Geometry check sheet. Reference: the model listing, model coordinates, mm. A direction names the side the tool comes from. Round coordinates to 2 decimals unless told otherwise and drop trailing zeros. Write each loop counter-clockwise with the first axis right and the second up, starting at its lowest first coordinate (ties: lowest second). Pieces come first, ordered by that corner, then holes. Notation, with made-up numbers: M 1,-13.5 L 39,-13.5 A25 ccw 39,19.5 Z; hole C 73,63 d2. An arc over 180 degrees is marked long. Use a Markdown table: item, result.
```python
from build123d import *
from build123d.topology import SkipClean

# Parameters (mm, degrees)
SKETCH_1_W            = 9.1
SKETCH_1_H            = 5.6
EXTRUDE_1_DEPTH       = 1.78
SKETCH_2_W            = 6.1
SKETCH_2_H            = 5.6
EXTRUDE_2_DEPTH       = 1.4
SWEEP_START           = -2.28
SWEEP_2_DEPTH         = 0.76
MIRROR_START          = -2.28
MIRROR_2_COPY_1_DEPTH = 0.76


# Read off the part's stored shape, not the designer's step: 스윕2
with BuildPart() as part:
    # 스케치1 → 보스-돌출1 (new body)
    with BuildSketch(Plane.XY):
        Rectangle(SKETCH_1_W, SKETCH_1_H)
    extrude(amount=EXTRUDE_1_DEPTH)

    # 스케치2 → 보스-돌출2 (add)
    with BuildSketch(Plane.XY.offset(1.78)):
        Rectangle(SKETCH_2_W, SKETCH_2_H)
    extrude(amount=EXTRUDE_2_DEPTH)

    # 스케치3 → 회전1 (revolve)
    with SkipClean():  # the faces are left unmerged after this step: merging them gives an invalid solid
        with BuildSketch(Plane(origin=(0, 0, 0), x_dir=(1, 0, 0), z_dir=(0, 1, 0))):
            with BuildLine():
                Line((-0.579062876, -3.18), (0.579062876, -3.18))
                ThreePointArc((0.579062876, -3.18), (0, -3.759062876), (-0.579062876, -3.18))
            make_face()
        revolve(axis=Axis((-0.579062876, 0, 3.18), (1, 0, 0)))

    # 스윕2 outline → 스윕2 (add)
    with SkipClean():  # the faces are left unmerged after this step: merging them gives an invalid solid
        with BuildSketch(Plane(origin=(0, 0, 0), x_dir=(1, 0, 0), z_dir=(0, 1, 0)).offset(SWEEP_START)):
            with BuildLine():
                Line((6.848797328, -0.399996384), (6.851202672, -3.616e-06))
                Line((6.851202672, -3.616e-06), (6.043424326, 0.004853607))
                ThreePointArc((6.043424326, 0.004853607), (5.654230205, -0.155982007), (5.492969053, -0.545))
                ThreePointArc((5.492969053, -0.545), (5.450499536, -0.647530483), (5.347969053, -0.69))
                Line((5.347969053, -0.69), (4.55, -0.69))
                Line((4.55, -0.69), (4.55, -1.09))
                Line((4.55, -1.09), (5.347969053, -1.09))
                ThreePointArc((5.347969053, -1.09), (5.733342249, -0.930373196), (5.892969053, -0.545))
                ThreePointArc((5.892969053, -0.545), (5.936647868, -0.439250079), (6.042221667, -0.395147271))
                Line((6.042221667, -0.395147271), (6.848797328, -0.399996384))
            make_face()
        sweep_2 = extrude(amount=SWEEP_2_DEPTH)

    # 대칭 복사1: 스윕2 across plane
    with SkipClean():  # the faces are left unmerged after this step: merging them gives an invalid solid
        add(sweep_2.mirror(Plane.ZX))

    # 대칭 복사2: 스윕2 across plane
    with SkipClean():  # the faces are left unmerged after this step: merging them gives an invalid solid
        add(sweep_2.mirror(Plane(origin=(0, 0, 0), x_dir=(0, 0, 1), z_dir=(1, 0, 0))))

    # 대칭 복사2 copy 1 sketch → 대칭 복사2 copy 1 (add)
    with SkipClean():  # the faces are left unmerged after this step: merging them gives an invalid solid
        with BuildSketch(Plane(origin=(0, 0, 0), x_dir=(-1, 0, 0), z_dir=(0, -1, 0)).offset(MIRROR_START)):
            with BuildLine():
                Line((6.848797328, -0.399996384), (6.851202672, -3.616e-06))
                Line((6.851202672, -3.616e-06), (6.043424326, 0.004853607))
                ThreePointArc((6.043424326, 0.004853607), (5.654230205, -0.155982007), (5.492969053, -0.545))
                ThreePointArc((5.492969053, -0.545), (5.450499536, -0.647530483), (5.347969053, -0.69))
                Line((5.347969053, -0.69), (4.55, -0.69))
                Line((4.55, -0.69), (4.55, -1.09))
                Line((4.55, -1.09), (5.347969053, -1.09))
                ThreePointArc((5.347969053, -1.09), (5.733342249, -0.930373196), (5.892969053, -0.545))
                ThreePointArc((5.892969053, -0.545), (5.936647868, -0.439250079), (6.042221667, -0.395147271))
                Line((6.042221667, -0.395147271), (6.848797328, -0.399996384))
            make_face()
        extrude(amount=MIRROR_2_COPY_1_DEPTH)


solid = part.part
```
Item 1: Material ranges on line 1 along X through (y, z) = (0.85, 2.1); line 2 along Z through (x, y) = (3.25, 0.95); line 3 along Z through (x, y) = (1.5, -0.6), recorded low to high. Write a range as from..to.
Outcome:
| item | result |
|---|---|
| line 1 | x = -3.05..3.05 |
| line 2 | z = 0..1.78 |
| line 3 | z = 0..3.18 |
Item 2: Cross-section at A-A, the plane y = -2.05. Record the cut outline in (x, z) (3 decimals).
Outcome:
| item | result |
|---|---|
| outline | M -6.851,0 L -6.043,-0.005 A0.55 ccw -5.493,0.545 A0.145 cw -5.348,0.69 L -4.55,0.69 L -4.55,0 L 4.55,0 L 4.55,0.69 L 5.348,0.69 A0.145 cw 5.493,0.545 A0.55 ccw 6.043,-0.005 L 6.851,0 L 6.849,0.4 L 6.042,0.395 A0.15 cw 5.893,0.545 A0.545 ccw 5.348,1.09 L 4.55,1.09 L 4.55,1.78 L 3.05,1.78 L 3.05,3.18 L -3.05,3.18 L -3.05,1.78 L -4.55,1.78 L -4.55,1.09 L -5.348,1.09 A0.545 ccw -5.893,0.545 A0.15 cw -6.042,0.395 L -6.849,0.4 Z |
Item 3: Cross-section at D-D, the plane y = -0.2. Record the cut outline in (x, z), and give its area (3 significant figures).
Outcome:
| item | result |
|---|---|
| outline | M -4.55,0 L 4.55,0 L 4.55,1.78 L 3.05,1.78 L 3.05,3.18 L 0.54,3.18 A0.54 ccw -0.54,3.18 L -3.05,3.18 L -3.05,1.78 L -4.55,1.78 Z |
| area | 25.2 mm2 |
Item 4: Access from +Z, -Z, +X, -X, +Y, -Y to the whole of each face (thin tool, end or side, straight path). Record for faces 4 (the face through (-4, 0, 1.78)), 5 (the face through (-5.7, 2.28, 0.5)), 6 (the face through (-5.7, -1.52, 0.5)), 7 (the face through (-5.7, -2.28, 0.5)), 8 (the face through (5.7, -2.28, 0.5)).
Outcome:
| item | result |
|---|---|
| face 4 | +Z, -X, +Y, -Y |
| face 5 | +Z, -Z, -X, +Y |
| face 6 | +Z, -Z, -X |
| face 7 | +Z, -Z, -X, -Y |
| face 8 | +Z, -Z, +X, -Y |
Item 5: Cross-section at B-B, the plane x = 0.75. Record the cut outline in (y, z), and give its area (3 significant figures).
Outcome:
| item | result |
|---|---|
| outline | M -2.8,0 L 2.8,0 L 2.8,3.18 L -2.8,3.18 Z |
| area | 17.8 mm2 |
Item 6: Mould release check, pull along Y, two halves, no side actions. Record for faces 1 (the face through (-3.05, 0, 2)), 2 (the face through (5.7, -1.52, 0.5)), 3 (the face through (5.7, 2.28, 0.5)): +Y half, -Y half, draft (parallel to the pull), parting line (faces both ways), or undercut.
Outcome:
| item | result |
|---|---|
| face 1 | draft |
| face 2 | undercut |
| face 3 | +Y half |
Item 7: Cross-section at C-C, the plane z = 1.25. Record the cut outline in (x, y), and give its area (3 significant figures).
Outcome:
| item | result |
|---|---|
| outline | M -4.55,-2.8 L 4.55,-2.8 L 4.55,2.8 L -4.55,2.8 Z |
| area | 51.0 mm2 |
Item 8: Go/stop test with flat-tipped pins: pin 1 (1.2 mm diameter, centred on x = -5.5, z = 0.5, fed in from +Y); pin 2 (1.6 mm diameter, centred on x = -4, y = 0, fed in from +Z); pin 3 (0.9 mm diameter, centred on x = 6, z = 0.5, fed in from -Y); pin 4 (2 mm diameter, centred on y = 1.5, z = 1, fed in from +X). Record where each tip stops, or that it passes through.
Outcome:
| item | result |
|---|---|
| pin 1 | stops at y = 2.28 |
| pin 2 | stops at z = 1.78 |
| pin 3 | stops at y = -2.28 |
| pin 4 | stops at x = 6.85 |
